```python
from build123d import *

# Parameters (mm, degrees)
SKETCH1_W           = 26
SKETCH1_H           = 10
BOSS_EXTRUDE1_DEPTH = 2.5
FILLET1_SIZE        = 3
SKETCH4_5_R         = 2.25
SKETCH3_6_R         = 4


with BuildPart() as part:
    # Sketch1 → Boss-Extrude1 (new body)
    with BuildSketch(Plane(origin=(0, 0, 0), x_dir=(0, 0, -1), z_dir=(1, 0, 0))):
        with Locations((13, 5)):
            Rectangle(SKETCH1_W, SKETCH1_H)
    extrude(amount=BOSS_EXTRUDE1_DEPTH)

    # Fillet1
    # a fillet whose section is not a circle: 3 mm, written as the material it takes off along each edge
    with BuildSketch(Plane(origin=(-7.5, 10, 0), x_dir=(0, 0, -1), z_dir=(1, 0, 0)), Plane(origin=(-7.5, 0, -26), x_dir=(0, 0, 1), z_dir=(1, 0, 0)), Plane(origin=(-7.5, 10, -26), x_dir=(0, -1, 0), z_dir=(1, 0, 0))) as fillet1_piece_1:
        with BuildLine():
            add(Edge.make_bspline([(FILLET1_SIZE, 0), (FILLET1_SIZE * 0.831801948466, 0), (FILLET1_SIZE * 0.663603896932, 0), (FILLET1_SIZE * 0.292893218813, -FILLET1_SIZE * 0.0716919198361), (FILLET1_SIZE * 0.0716919198361, -FILLET1_SIZE * 0.292893218813), (0, -FILLET1_SIZE * 0.663603896932), (0, -FILLET1_SIZE * 0.831801948466), (0, -FILLET1_SIZE)], knots=[0, 0, 0, 0, 0, 0, 0.5, 0.5, 1, 1, 1, 1, 1, 1], degree=5))
            Line((0, -FILLET1_SIZE), (0, 0))
            Line((0, 0), (FILLET1_SIZE, 0))
        make_face()
    extrude(amount=17.5, mode=Mode.SUBTRACT)
    with BuildSketch(Plane(origin=(-7.5, 0, 0), x_dir=(0, 0, -1), z_dir=(1, 0, 0))) as fillet1_piece_2:
        with BuildLine():
            add(Edge.make_bspline([(FILLET1_SIZE, 0), (FILLET1_SIZE * 0.831801948466, 0), (FILLET1_SIZE * 0.663603896932, 0), (FILLET1_SIZE * 0.292893218813, FILLET1_SIZE * 0.0716919198361), (FILLET1_SIZE * 0.0716919198361, FILLET1_SIZE * 0.292893218813), (0, FILLET1_SIZE * 0.663603896932), (0, FILLET1_SIZE * 0.831801948466), (0, FILLET1_SIZE)], knots=[0, 0, 0, 0, 0, 0, 0.5, 0.5, 1, 1, 1, 1, 1, 1], degree=5))
            Line((0, FILLET1_SIZE), (0, 0))
            Line((0, 0), (FILLET1_SIZE, 0))
        make_face()
    extrude(amount=17.5, mode=Mode.SUBTRACT)

    # Cut-Loft1: read off the stored shape, not the designer's step
    # Cut-Loft1: loft between two sections, ruled curve by curve
    cut_loft1_from = [
        Edge.make_bspline([(0, 5.227220393, -4.761502537), (0, 5.040678937, -4.742567504), (0, 4.827360743, -4.743831636), (0, 4.355343831, -4.831009815), (0, 4.09562853, -4.918026839), (0, 3.710202489, -5.150291271), (0, 3.582651152, -5.2453356), (0, 3.342613634, -5.469976954), (0, 3.230127455, -5.599573979), (0, 3.033437391, -5.892627716), (0, 2.949592094, -6.055325315), (0, 2.823029016, -6.402187173), (0, 2.780437569, -6.586238152), (0, 2.742567504, -6.959321063), (0, 2.747306812, -7.148176386), (0, 2.801589604, -7.513395142), (0, 2.851032094, -7.68962222), (0, 2.984823778, -8.016221759), (0, 3.068974238, -8.165778536), (0, 3.258976095, -8.434071364), (0, 3.364827492, -8.552807416), (0, 3.695720639, -8.857782374), (0, 3.932653309, -8.995212029), (0, 4.377524958, -9.175459681), (0, 4.586238152, -9.219562431), (0, 4.959321063, -9.257432496), (0, 5.172639257, -9.256168364), (0, 5.644656169, -9.168990185), (0, 5.90437147, -9.081973161), (0, 6.289797511, -8.849708729), (0, 6.417348848, -8.7546644), (0, 6.657386366, -8.530023046), (0, 6.769872545, -8.400426021), (0, 6.966562609, -8.107372284), (0, 7.050407906, -7.944674685), (0, 7.176970984, -7.597812827), (0, 7.219562431, -7.413761848), (0, 7.257432496, -7.040678937), (0, 7.252693188, -6.851823614), (0, 7.198410396, -6.486604858), (0, 7.148967906, -6.31037778), (0, 7.015176222, -5.983778241), (0, 6.931025762, -5.834221464), (0, 6.741023905, -5.565928636), (0, 6.635172508, -5.447192584), (0, 6.304279361, -5.142217626), (0, 6.067346691, -5.004787971), (0, 5.622475042, -4.824540319), (0, 5.413761848, -4.780437569), (0, 5.227220393, -4.761502537)], [0, 0, 0, 0, 0.0625, 0.0625, 0.125, 0.125, 0.15625, 0.15625, 0.1875, 0.1875, 0.21875, 0.21875, 0.25, 0.25, 0.28125, 0.28125, 0.3125, 0.3125, 0.34375, 0.34375, 0.375, 0.375, 0.4375, 0.4375, 0.5, 0.5, 0.5625, 0.5625, 0.625, 0.625, 0.65625, 0.65625, 0.6875, 0.6875, 0.71875, 0.71875, 0.75, 0.75, 0.78125, 0.78125, 0.8125, 0.8125, 0.84375, 0.84375, 0.875, 0.875, 0.9375, 0.9375, 1, 1, 1, 1], 3),
    ]
    cut_loft1_to = [
        Edge.make_bspline([(2.5, 2.811561531, -3.602638399), (2.5, 2.528448064, -3.778586903), (2.5, 2.229585449, -4.012046448), (2.5, 1.65992568, -4.647393225), (2.5, 1.388895654, -5.051936935), (2.5, 1.098683643, -5.797441454), (2.5, 1.021967094, -6.068450115), (2.5, 0.927996054, -6.645321276), (2.5, 0.910956437, -6.951185481), (2.5, 0.952403615, -7.577266038), (2.5, 1.011097599, -7.897318025), (2.5, 1.209685139, -8.522967618), (2.5, 1.349633474, -8.828268581), (2.5, 1.701530482, -9.394495515), (2.5, 1.913312576, -9.655153449), (2.5, 2.386369409, -10.110226694), (2.5, 2.647353909, -10.30455978), (2.5, 3.19037235, -10.618925341), (2.5, 3.472167179, -10.739070815), (2.5, 4.031019985, -10.910226979), (2.5, 4.307984356, -10.961431088), (2.5, 5.104928058, -11.031293352), (2.5, 5.587659325, -10.967391766), (2.5, 6.409558868, -10.737916455), (2.5, 6.75121216, -10.573310105), (2.5, 7.317439093, -10.221413097), (2.5, 7.616301709, -9.987953552), (2.5, 8.185961477, -9.352606775), (2.5, 8.456991504, -8.948063065), (2.5, 8.747203514, -8.202558546), (2.5, 8.823920064, -7.931549885), (2.5, 8.917891104, -7.354678724), (2.5, 8.934930721, -7.048814519), (2.5, 8.893483543, -6.422733962), (2.5, 8.834789558, -6.102681975), (2.5, 8.636202018, -5.477032382), (2.5, 8.496253684, -5.171731419), (2.5, 8.144356676, -4.605504485), (2.5, 7.932574581, -4.344846551), (2.5, 7.459517749, -3.889773306), (2.5, 7.198533248, -3.69544022), (2.5, 6.655514807, -3.381074659), (2.5, 6.373719979, -3.260929185), (2.5, 5.814867172, -3.089773021), (2.5, 5.537902802, -3.038568912), (2.5, 4.7409591, -2.968706648), (2.5, 4.258227833, -3.032608234), (2.5, 3.436328289, -3.262083545), (2.5, 3.094674998, -3.426689895), (2.5, 2.811561531, -3.602638399)], [0, 0, 0, 0, 0.0625, 0.0625, 0.125, 0.125, 0.15625, 0.15625, 0.1875, 0.1875, 0.21875, 0.21875, 0.25, 0.25, 0.28125, 0.28125, 0.3125, 0.3125, 0.34375, 0.34375, 0.375, 0.375, 0.4375, 0.4375, 0.5, 0.5, 0.5625, 0.5625, 0.625, 0.625, 0.65625, 0.65625, 0.6875, 0.6875, 0.71875, 0.71875, 0.75, 0.75, 0.78125, 0.78125, 0.8125, 0.8125, 0.84375, 0.84375, 0.875, 0.875, 0.9375, 0.9375, 1, 1, 1, 1], 3),
    ]
    cut_loft1 = Solid(Shell([*[Face.make_surface_from_curves(cut_loft1_from[k], cut_loft1_to[k]) for k in range(1)], Face(Wire(cut_loft1_from)), Face(Wire(cut_loft1_to))]))
    add(cut_loft1, mode=Mode.SUBTRACT)

    # Sketch4<5> → Cut-Loft2 section 0
    with BuildSketch(Plane.ZY):
        with Locations((-19, 5)):
            Circle(SKETCH4_5_R)
    # Sketch3<6> → Cut-Loft2 section 1
    with BuildSketch(Plane(origin=(2.5, 0, 0), x_dir=(0, 0, -1), z_dir=(1, 0, 0))):
        with Locations((19, 5.077056421)):
            Circle(SKETCH3_6_R)
    loft(mode=Mode.SUBTRACT)


solid = part.part
```
Geometry check sheet. Reference: the model listing, model coordinates, mm. Coordinates: 2 decimals unless noted, no trailing zeros.
Item 1: Thickness scan on line 1 (Z direction, x = 2, y = 7); line 2 (Z direction, x = 1.9, y = 4.25); line 3 (Y direction, x = 2.2, z = -18.25). Record the ranges inside material, lowest first.
Item 2: Sectioned sample at A-A, the plane x = 0.3. Count the separate pieces of the cut face and the enclosed holes in it, then the cut area to 3 significant figures.
Item 3: Go/stop test with flat-tipped pins: pin 1 Ø1.5 at (x, z) = (0.5, -17) entering from -Y; pin 2 Ø1.5 at (x, y) = (2, 8.5) entering from -Z. Record where each tip stops, or that it passes through.
Check result:
1. line 1: z = -26 to -22.09, -15.91 to -9.91, -4.09 to 0
1. line 2: z = -26 to -22.49, -15.51 to -10.41, -3.59 to 0
1. line 3: y = 0 to 1.35, 8.78 to 10
2. separate pieces: 1
2. enclosed holes: 2
2. area: 218 mm2
3. pin 1: stops at y = 0
3. pin 2: stops at z = -25.98
